```python
from build123d import *

# Parameters (mm, degrees)
F1_DEPTH      = 49.8856
F2_W          = 4.8768
F2_H          = 4.8768
F3_DEPTH      = 25.4
F3_DEPTH_BACK = 25.4
F2_R          = 6.096
F4_DEPTH      = 8.7386
F4_DEPTH_BACK = 3.175


with BuildPart() as f1:
    # F0 (on Front) → F1 (new body)
    with BuildSketch(Plane.XZ):
        with BuildLine():
            Line((-21.971, 5.567192), (-21.971, -3.175))
            Line((-21.971, -3.175), (-18.796, -3.175))
            Line((-18.796, -3.175), (-18.796, -1.651))
            Line((-18.796, -1.651), (-14.4272, -1.651))
            Line((-14.4272, -1.651), (-14.4272, -6.35))
            Line((-14.4272, -6.35), (0, -6.35))
            Line((0, -6.35), (14.4272, -6.35))
            Line((14.4272, -6.35), (14.4272, -1.651))
            Line((14.4272, -1.651), (18.796, -1.651))
            Line((18.796, -1.651), (18.796, -3.175))
            Line((18.796, -3.175), (21.971, -3.175))
            Line((21.971, -3.175), (21.971, 5.567192))
            ThreePointArc((21.971, 5.567192), (19.888745, 8.545012), (16.37714, 7.611298))
            ThreePointArc((16.37714, 7.611298), (9.029709, 1.99578), (0, 0))
            ThreePointArc((0, 0), (-9.029709, 1.99578), (-16.37714, 7.611298))
            ThreePointArc((-16.37714, 7.611298), (-19.888745, 8.545012), (-21.971, 5.567192))
        make_face()
    extrude(amount=F1_DEPTH)

    # F2 (on Top) → F3 (cut, two sides)
    with BuildSketch(Plane.XY) as f3_sk:
        with Locations((0, -9.525)):
            Rectangle(F2_W, F2_H)
        with Locations((0, -40.3606)):
            Rectangle(F2_W, F2_H)
    extrude(amount=F3_DEPTH, mode=Mode.SUBTRACT)
    extrude(f3_sk.sketch, amount=-F3_DEPTH_BACK, mode=Mode.SUBTRACT)

    # F2 (on Top) → F4 (cut, two sides)
    with BuildSketch(Plane.XY) as f4_sk:
        with Locations((0, -40.3606)):
            Circle(F2_R)
        with Locations((0, -40.3606)):
            Rectangle(F2_W, F2_H, mode=Mode.SUBTRACT)
        with Locations((0, -9.525)):
            Circle(F2_R)
        with Locations((0, -9.525)):
            Rectangle(F2_W, F2_H, mode=Mode.SUBTRACT)
        with Locations((0, -40.3606)):
            Rectangle(F2_W, F2_H)
        with Locations((0, -9.525)):
            Rectangle(F2_W, F2_H)
    extrude(amount=F4_DEPTH, mode=Mode.SUBTRACT)
    extrude(f4_sk.sketch, amount=-F4_DEPTH_BACK, mode=Mode.SUBTRACT)


solid = f1.part
```
Design review of the part built by this model. Coordinates are the model's own, in mm. A direction names the side the tool comes from. Coordinates: 2 decimals unless noted, no trailing zeros. Order: outer loops, then holes, each group sorted by start corner. A loop starts at its lowest first (then second) coordinate and runs counter-clockwise, first axis right, second up. Notation, with made-up numbers: (-28.75, 15.25) - (1.25, 15.25) arc R20 ccw to (1.25, 27.25) - close; hole circle Ø10 at (60.25, 33). An arc over 180 degrees is marked (long way). Answer in a Markdown table with one row per item.
(1) The part is to be moulded in two halves that separate along X. For faces 6 (the flat face through (-0.3, 0, -0.4)), 7 (the flat face through (-21.971, -25, 1)), 8 (the flat face through (-14.427, -25, -4)), say which applies: released by +X, released by -X, zero draft, split by the parting line, or undercut.
Checked values:
| item | result |
|---|---|
| face 6 | zero draft |
| face 7 | released by -X |
| face 8 | undercut |
(2) Consider section C-C on z = -4.25. State the section outline as (x, y) points, plus the area to 3 significant figures.
Checked values:
| item | result |
|---|---|
| outline | (-14.43, -49.89) - (14.43, -49.89) - (14.43, 0) - (-14.43, 0) - close; hole (-2.44, -42.8) - (2.44, -42.8) - (2.44, -37.92) - (-2.44, -37.92) - close; hole (-2.44, -11.96) - (2.44, -11.96) - (2.44, -7.09) - (-2.44, -7.09) - close |
| area | 1,390 mm^2 |
(3) Consider section D-D on y = -26.5. State the section outline as (x, z) points (3 decimals), plus the area to 3 significant figures.
Checked values:
| item | result |
|---|---|
| outline | (-21.971, -3.175) - (-18.796, -3.175) - (-18.796, -1.651) - (-14.427, -1.651) - (-14.427, -6.35) - (14.427, -6.35) - (14.427, -1.651) - (18.796, -1.651) - (18.796, -3.175) - (21.971, -3.175) - (21.971, 5.567) arc R3.17 ccw to (16.377, 7.611) arc R21.425 cw to (0, 0) arc R21.425 cw to (-16.377, 7.611) arc R3.17 ccw to (-21.971, 5.567) - close |
| area | 386 mm^2 |
(4) For faces 1 (the flat face through (0, -25, -6.35)), 2 (the flat face through (-18.796, -25, -2)), 3 (the flat face through (21.971, -25, 1)), 4 (the flat face through (-20, -25, -3.175)), 5 (the flat face through (0, -37.922, -5)), list the 3-axis set-ups (+Z, -Z, +X, -X, +Y, -Y) from which the entire face can be reached by the end or side of a thin tool; tool diameter is ignored.
Checked values:
| item | result |
|---|---|
| face 1 | -Z, +X, -X, +Y, -Y |
| face 2 | -Z, +Y, -Y |
| face 3 | +Z, -Z, +X, +Y, -Y |
| face 4 | -Z, -X, +Y, -Y |
| face 5 | +Z, -Z |
(5) Consider section B-B on x = 1. State the section outline as (y, z) points (3 decimals).
Checked values:
| item | result |
|---|---|
| outline | (-49.886, -6.35) - (-42.799, -6.35) - (-42.799, -3.175) - (-46.374, -3.175) - (-46.374, 0.023) - (-49.886, 0.023) - close; (-37.922, -6.35) - (-11.963, -6.35) - (-11.963, -3.175) - (-15.538, -3.175) - (-15.538, 0.023) - (-34.347, 0.023) - (-34.347, -3.175) - (-37.922, -3.175) - close; (-7.087, -6.35) - (0, -6.35) - (0, 0.023) - (-3.512, 0.023) - (-3.512, -3.175) - (-7.087, -3.175) - close |
(6) Clearance check with flat-ended pins moving along their axes: pin 1 (1 mm diameter, centred on x = 0, z = -5, fed in from +Y); pin 2 (1.6 mm diameter, centred on x = -20, y = -20, fed in from -Z) (3 decimals); pin 3 (4 mm diameter, centred on x = 0.5, y = -27, fed in from +Z); pin 4 (3.5 mm diameter, centred on y = -10, z = -5.5, fed in from +X). State where each tip first meets the part, or that it passes through.
Checked values:
| item | result |
|---|---|
| pin 1 | y = 0 |
| pin 2 | z = -3.175 |
| pin 3 | z = 0.15 |
| pin 4 | x = 14.43 |
(7) Consider section A-A on z = 2.5. State the section outline as (x, y) points.
Checked values:
| item | result |
|---|---|
| outline | (-21.97, -49.89) - (-10.04, -49.89) - (-10.04, 0) - (-21.97, 0) - close; (10.04, -49.89) - (21.97, -49.89) - (21.97, 0) - (10.04, 0) - close |
(8) Wall thickness on line 1 along Y through (x, z) = (0, -1.6); line 2 along Y through (x, z) = (5.5, -0.5); line 3 along X through (y, z) = (-22, 5.75): over which ranges is each line inside the solid? List them lowest first. Write a range as from..to.
Checked values:
| item | result |
|---|---|
| line 1 | -49.89..-46.46, -34.26..-15.62, -3.43..0 |
| line 2 | -49.89..-42.99, -37.73..-12.15, -6.9..0 |
| line 3 | -21.97..-14.61, 14.61..21.97 |
